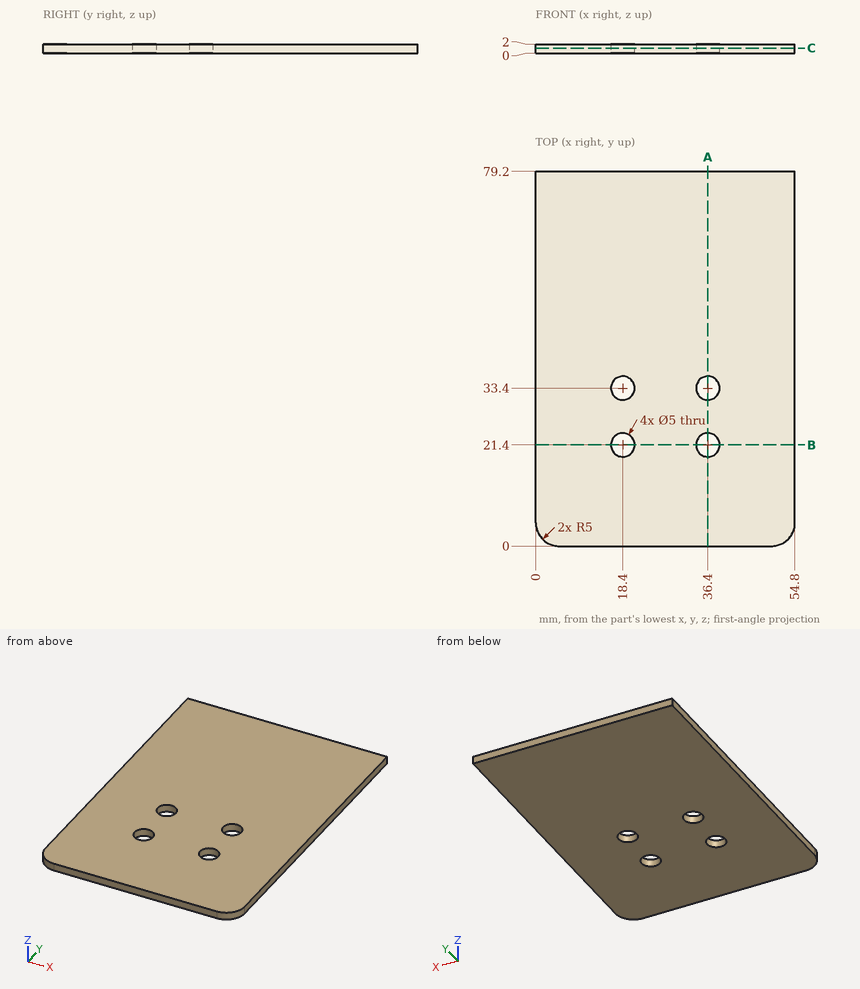
Study the drawing (mm; zero at the part's minimum x, y, z) and answer. Round coordinates to 2 decimals unless told otherwise and drop trailing zeros. Write each loop counter-clockwise with the first axis right and the second up, starting at its lowest first coordinate (ties: lowest second). Pieces come first, ordered by that corner, then holes. Notation, with made-up numbers: (47.25, 67.5) -> (83.25, 67.5) arc R30 cw to (83.25, 105.5) -> close; hole circle Ø5 at (55.5, -32.5). An arc over 180 degrees is marked (long way). Write item = value, one per line.
1) Section C-C on z = 1.15 is taken. Write down the section's boundary in (x, y), plus the area to 3 significant figures.
Check values:
outline = (0, 5) arc R5 ccw to (5, 0) -> (49.8, 0) arc R5 ccw to (54.8, 5) -> (54.8, 79.2) -> (0, 79.2) -> close; hole circle Ø5 at (18.4, 21.4); hole circle Ø5 at (18.4, 33.4); hole circle Ø5 at (36.4, 21.4); hole circle Ø5 at (36.4, 33.4)
area = 4,250 mm²
2) A straight line is drawn through the part: line 1 along Y through (x, z) = (36.4, 1.05). Find the intervals that lie inside material, in ascending order. Write a range as [from, to].
Check values:
line_1 = [0, 18.9], [23.9, 30.9], [35.9, 79.2]
3) Section B-B on y = 21.4 is taken. Write down the section's boundary in (x, z), plus the area to 3 significant figures.
Check values:
outline = (0, 0) -> (15.9, 0) -> (15.9, 2) -> (0, 2) -> close; (20.9, 0) -> (33.9, 0) -> (33.9, 2) -> (20.9, 2) -> close; (38.9, 0) -> (54.8, 0) -> (54.8, 2) -> (38.9, 2) -> close
area = 89.6 mm²
4) Section A-A on x = 36.4 is taken. Write down the section's boundary in (y, z).
Check values:
outline = (0, 0) -> (18.9, 0) -> (18.9, 2) -> (0, 2) -> close; (23.9, 0) -> (30.9, 0) -> (30.9, 2) -> (23.9, 2) -> close; (35.9, 0) -> (79.2, 0) -> (79.2, 2) -> (35.9, 2) -> close
